For this review, use the dimensioned drawing (mm, ordinates from the lowest corner) and the shaded views. A direction names the side the tool comes from. Round coordinates to 2 decimals unless told otherwise and drop trailing zeros. Loops run counter-clockwise (first coordinate to the right, second up) from the corner with the lowest first, then second, coordinate; pieces in that order, holes last. Notation, with made-up numbers: M 23,29.25 L 58,29.25 A26 cw 58,56.25 Z; hole C -5.5,-17 d10. An arc over 180 degrees is marked long. Answer as a JSON object with one key per item and string values. Group by question number.
Item 1: Consider section D-D (y = 14). Give the boundary of the cut face in (x, z), and give its area (3 significant figures).
Item 2: Insertion check: P1, Ø1.5, axis at y = 8, z = 9.5, coming from the +X side; P2, Ø7.5, axis at y = 10, z = 12.5, coming from the -X side; P3, Ø3, axis at x = 25, y = 7.5, coming from the +Z side; P4, Ø8, axis at x = 3, y = 4, coming from the -Z side. Each pin has a flat end and moves straight along its axis. Give the tip position at first contact, or say it passes through.
Item 3: Consider section C-C (y = 7.5). Give the boundary of the cut face in (x, z).
Item 4: Consider section A-A (x = 6.5). Give the boundary of the cut face in (y, z), and give its area (4 significant figures).
Item 5: Consider section B-B (z = 26.5). Give the boundary of the cut face in (x, y).
Item 6: Tool access review of the marked faces 1, 2 and 3: name each direction out of +Z, -Z, +X, -X, +Y, -Y from which nothing blocks a thin tool from reaching the whole face with its end or side.
Item 7: To check wall thickness, follow line 1 (Z direction, x = 6.5, y = 10.75); line 2 (Y direction, x = 25, z = 0.7); line 3 (X direction, y = 11.75, z = 7). State the ranges of each line that lie inside material, in increasing order.
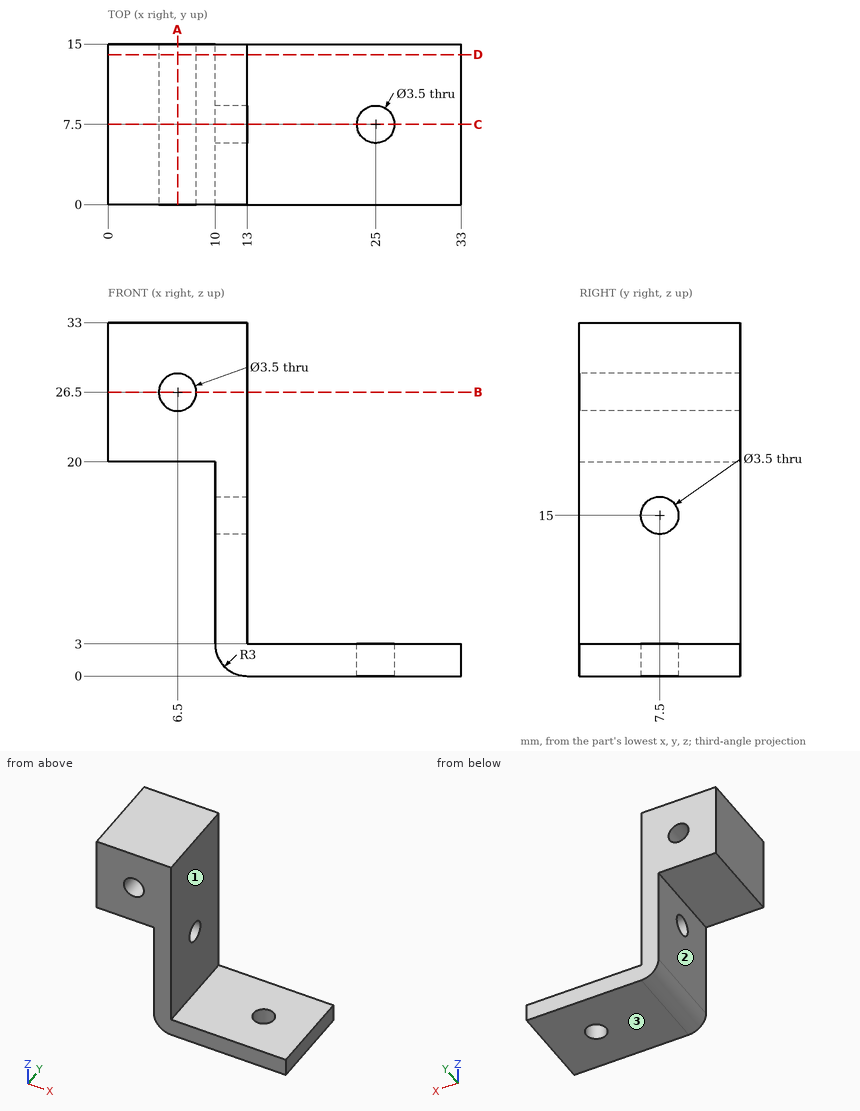
Geometry results:
{
 "1": {"outline": "M 0,20 L 10,20 L 10,3 A3 ccw 13,0 L 33,0 L 33,3 L 13,3 L 13,33 L 0,33 Z; hole C 6.5,26.5 d3.5", "area": "277 mm^2"},
 "2": {"P1": "stops at x = 13", "P2": "stops at x = 10", "P3": "passes through", "P4": "stops at z = 20"},
 "3": {"outline": "M 0,20 L 10,20 L 10,16.75 L 13,16.75 L 13,33 L 0,33 Z; M 10,3 A3 ccw 13,0 L 23.25,0 L 23.25,3 L 13,3 L 13,13.25 L 10,13.25 Z; M 26.75,0 L 33,0 L 33,3 L 26.75,3 Z; hole C 6.5,26.5 d3.5"},
 "4": {"outline": "M 0,20 L 15,20 L 15,24.75 L 0,24.75 Z; M 0,28.25 L 15,28.25 L 15,33 L 0,33 Z", "area": "142.5 mm^2"},
 "5": {"outline": "M 0,0 L 4.75,0 L 4.75,15 L 0,15 Z; M 8.25,0 L 13,0 L 13,15 L 8.25,15 Z"},
 "6": {"face 1": "+Z, +X, +Y, -Y", "face 2": "-Z, -X, +Y, -Y", "face 3": "-Z, +X, -X, +Y, -Y"},
 "7": {"line 1": "z = 20 to 24.75, 28.25 to 33", "line 2": "y = 0 to 5.75, 9.25 to 15", "line 3": "x = 10 to 13"}
}
